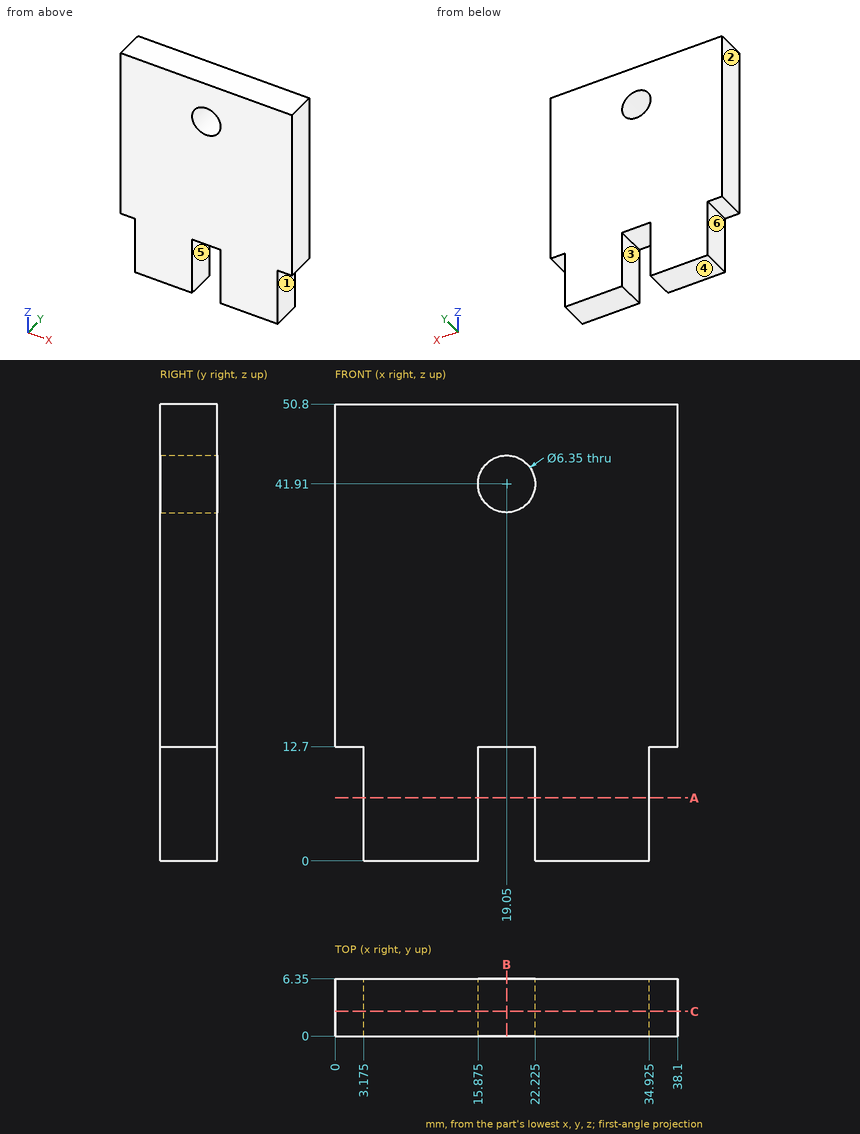
Part print with two shaded views. Sizes in mm from the minimum x, y, z corner. A direction names the side the tool comes from. Round coordinates to 2 decimals unless told otherwise and drop trailing zeros. Order: outer loops, then holes, each group sorted by start corner. A loop starts at its lowest first (then second) coordinate and runs counter-clockwise, first axis right, second up. Notation, with made-up numbers: (87.5, 55) - (124.5, 55) arc R31 ccw to (124.5, 81) - close; hole circle Ø3 at (12, -8). An arc over 180 degrees is marked (long way). Return JSON: item names as keys, results as strings.
(1) Cut at B-B (x = 19.05). Give the cut face in (y, z) (3 decimals).
Answer key:
{"outline": "(0, 12.7) - (6.35, 12.7) - (6.35, 38.735) - (0, 38.735) - close; (0, 45.085) - (6.35, 45.085) - (6.35, 50.8) - (0, 50.8) - close"}
(2) Cut at C-C (y = 2.75). Give the cut face in (x, z) (3 decimals).
Answer key:
{"outline": "(0, 12.7) - (3.175, 12.7) - (3.175, 0) - (15.875, 0) - (15.875, 12.7) - (22.225, 12.7) - (22.225, 0) - (34.925, 0) - (34.925, 12.7) - (38.1, 12.7) - (38.1, 50.8) - (0, 50.8) - close; hole circle Ø6.35 at (19.05, 41.91)"}
(3) Tool access for the marked faces 4, 5 and 6: list every direction of +Z, -Z, +X, -X, +Y, -Y with a clear straight run to the whole face (end or side of a thin tool).
Answer key:
{"face 4": "-Z, +X, -X, +Y, -Y", "face 5": "-Z, +Y, -Y", "face 6": "-Z, -X, +Y, -Y"}
(4) Cut at A-A (z = 7). Give the cut face in (x, y) (3 decimals), then the cut area to 3 significant figures.
Answer key:
{"outline": "(3.175, 0) - (15.875, 0) - (15.875, 6.35) - (3.175, 6.35) - close; (22.225, 0) - (34.925, 0) - (34.925, 6.35) - (22.225, 6.35) - close", "area": "161 mm^2"}
(5) Pull direction X, two halves, no side cores. Call the marked faces 1, 2 and 3: +X half, -X half, draft (parallel to the pull), parting line (faces both ways), or undercut.
Answer key:
{"face 1": "+X half", "face 2": "-X half", "face 3": "undercut"}
(6) Pin check, flat tips, straight feed: pin 1 Ø3 at (x, y) = (18, 4.5) entering from -Z; pin 2 Ø1.9 at (y, z) = (4, 5.5) entering from +X (3 decimals). Stop position of each tip, or through.
Answer key:
{"pin 1": "stops at z = 12.7", "pin 2": "stops at x = 34.925"}
(7) Wall check: probe 1 along Z at (x, y) = (19.05, 1.5) (3 decimals); probe 2 along X at (y, z) = (5.5, 41.5); probe 3 along Z at (x, y) = (21.5, 3.25). Give the ranges that are in metal, low to high. Write a range as from..to.
Answer key:
{"probe 1": "z = 12.7..38.735, 45.085..50.8", "probe 2": "x = 0..15.9, 22.2..38.1", "probe 3": "z = 12.7..39.89, 43.93..50.8"}
